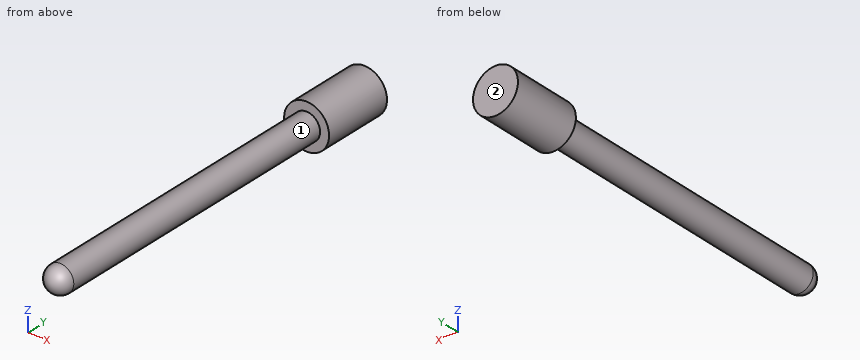
from build123d import *

# Parameters (mm, degrees)
SKETCH1_R           = 7.9375
BOSS_EXTRUDE1_DEPTH = 25.4
SKETCH2_R           = 4.7625
BOSS_EXTRUDE2_DEPTH = 107.95
DOME1_FACE_RADIUS   = 4.7625
DOME1_HEIGHT        = 4.7625


with BuildPart() as part:
    # Sketch1 → Boss-Extrude1 (new body)
    with BuildSketch(Plane(origin=(0, 0, 0), x_dir=(1, 0, 0), z_dir=(0, 1, 0))):
        with Locations(Location((0, 0, 0), (0, 0, 270))):  # turned: the seam where the file's is
            Circle(SKETCH1_R)
    extrude(amount=BOSS_EXTRUDE1_DEPTH)

    # Sketch2 → Boss-Extrude2 (add)
    with BuildSketch(Plane.XZ):
        with Locations(Location((0, 0, 0), (0, 0, 90))):  # turned: the seam where the file's is
            Circle(SKETCH2_R)
    extrude(amount=BOSS_EXTRUDE2_DEPTH)

    # Dome1: a dome of height H over a round flat face of radius A is a cap of a sphere of radius (A * A + H * H) / (2 * H)
    dome1_r = (DOME1_FACE_RADIUS * DOME1_FACE_RADIUS + DOME1_HEIGHT * DOME1_HEIGHT) / (2 * DOME1_HEIGHT)
    dome1_base = Plane((0, -107.95, 0), z_dir=(0, -1, 0))
    with Locations(dome1_base.offset(DOME1_HEIGHT - dome1_r)):
        dome1_ball = Sphere(dome1_r, mode=Mode.PRIVATE)
    add(split(dome1_ball, bisect_by=dome1_base, keep=Keep.TOP, mode=Mode.PRIVATE))


solid = part.part
Can you work these out from the model? Positions are in its coordinate system, mm. Face numbers are marked on the shaded views. A direction names the side the tool comes from. Give positions to 0.01 mm unless a question says otherwise; leave off trailing zeros. Loops run counter-clockwise (first coordinate to the right, second up) from the corner with the lowest first, then second, coordinate; pieces in that order, holes last. Notation, with made-up numbers: (22, 47) - (40, 47) arc R22 cw to (40, 68) - close; hole circle Ø8 at (52, -19.75). An arc over 180 degrees is marked (long way). Return JSON: item names as keys, results as strings.
1. I want a section at C-C on y = -71. Please give me the cut outline in (x, z) (1 decimal).
Output values:
{"outline": "circle Ø9.5 at (0, 0)"}
2. If I drill on line 1 (Y direction, x = -1.75, z = -7); line 2 (X direction, y = -28, z = -0.25); line 3 (Z direction, x = -3.5, y = -52.5), over which ranges is the centre line in solid material (lowest first)?
Output values:
{"line 1": "y = 0 to 25.4", "line 2": "x = -4.76 to 4.76", "line 3": "z = -3.23 to 3.23"}
3. I want a section at D-D on x = -6.75. Please give me the cut outline in (y, z).
Output values:
{"outline": "(0, -4.18) - (25.4, -4.18) - (25.4, 4.18) - (0, 4.18) - close"}
4. I'm going to push flat-ended pins straight in: pin 1 Ø2 at (x, y) = (-2, -21.5) entering from -Z; pin 2 Ø8 at (x, z) = (-4, -3) entering from -Y; pin 3 Ø1 at (x, y) = (3.5, -73) entering from -Z. Where does each tip first touch, or does it pass through?
Output values:
{"pin 1": "stops at z = -4.66", "pin 2": "stops at y = -112.61", "pin 3": "stops at z = -3.7"}
5. For the marked faces 1 and 2, which set-ups out of +Z, -Z, +X, -X, +Y, -Y let a thin tool reach every point of the face, with its end or its side?
Output values:
{"face 1": "-Y", "face 2": "+Z, -Z, +X, -X, +Y"}
